For this review, take the finished solid that the model builds, in its own axes (mm). Give positions to 0.01 mm unless a question says otherwise; leave off trailing zeros. Write each loop counter-clockwise with the first axis right and the second up, starting at its lowest first coordinate (ties: lowest second). Pieces come first, ordered by that corner, then holes. Notation, with made-up numbers: M 68.5,7 L 108.5,7 A5 ccw 108.5,16 Z; hole C 78.25,-22.5 d9. An arc over 180 degrees is marked long. Use one line per item in the form item = value. Start each with the question number.
Q1. Consider section A-A on z = -2.75. Write out the cut boundary in (x, y).
Q2. Consider section C-C on y = 2. Write out the cut boundary in (x, z).
Q3. Consider section B-B on x = 31. Write out the cut boundary in (y, z), and give its area (3 significant figures).
Q4. For probe 1 along X at (y, z) = (8, 0); probe 2 along Y at (x, z) = (35, 0), list the stretches that pass through material, from the lowest coordinate up. Write a range as [from, to].
Q5. Clearance check with flat-ended pins moving along their axes: pin 1 Ø6 at (y, z) = (5, 2.5) entering from +X; pin 2 Ø0.6 at (x, y) = (-5.5, 10.5) entering from -Z; pin 3 Ø1.5 at (y, z) = (9, -1) entering from +X. State where each tip first meets the part, or that it passes through.
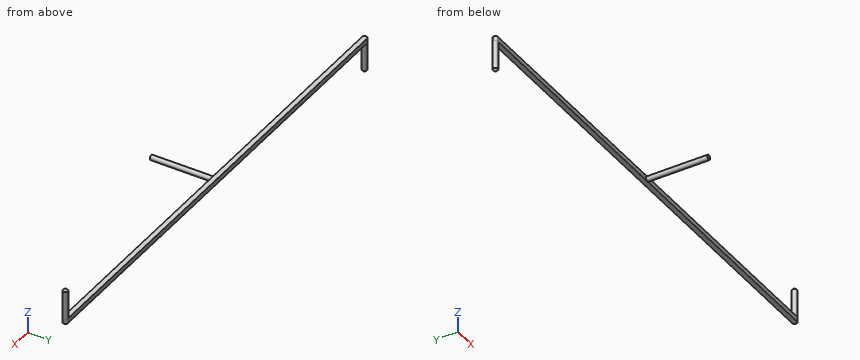
```python
from build123d import *

# Parameters (mm, degrees)
SKETCH_1_R      = 0.4
EXTRUDE_1_DEPTH = 10
SKETCH_2_W      = 80
SKETCH_2_H      = 0.8
EXTRUDE_2_DEPTH = 0.8
FILLET_1_R      = 0.4
SKETCH_3_R      = 0.4
EXTRUDE_3_DEPTH = 5
SKETCH_4_R      = 0.4
EXTRUDE_4_DEPTH = 5
CHAMFER_1_SIZE  = 0.4


with BuildPart() as part:
    # 草图1 → 凸台-拉伸1 (new body)
    with BuildSketch(Plane(origin=(0, 0, 0), x_dir=(1, 0, 0), z_dir=(0, 1, 0))):
        with Locations(Location((0, 0, 0), (0, 0, 270))):
            Circle(SKETCH_1_R)
    extrude(amount=EXTRUDE_1_DEPTH)

    # 草图2 → 凸台-拉伸2 (add)
    with BuildSketch(Plane(origin=(0, 10, 0), x_dir=(1, 0, 0), z_dir=(0, 1, 0))):
        Rectangle(SKETCH_2_W, SKETCH_2_H)
    extrude(amount=EXTRUDE_2_DEPTH)

    # 圆角1
    fillet_1_edges = [part.edges().sort_by_distance(p)[0] for p in [
        (40, 10, 0),
        (40, 10.8, 0),
        (-40, 10, 0),
        (-40, 10.8, 0),
    ]]
    fillet(fillet_1_edges, radius=FILLET_1_R - 0.0001)  # a hair under: the kernel refuses the full size

    # 草图3 → 凸台-拉伸3 (add)
    with BuildSketch(Plane.XY.offset(0.4)):
        with Locations((39.6, 10.4)):
            Circle(SKETCH_3_R)
    extrude(amount=EXTRUDE_3_DEPTH)

    # 草图4 → 凸台-拉伸4 (add)
    with BuildSketch(Plane(origin=(0, 0, -0.4), x_dir=(-1, 0, 0), z_dir=(0, 0, -1))):
        with Locations((39.6, 10.4)):
            Circle(SKETCH_4_R)
    extrude(amount=EXTRUDE_4_DEPTH)

    # 倒角1
    chamfer_1_edges = [part.edges().sort_by_distance(p)[0] for p in [
        (39.2, 10.4, 5.4),
        (-39.2, 10.4, -5.4),
    ]]
    chamfer(chamfer_1_edges, length=CHAMFER_1_SIZE - 0.0001)  # a hair under: the kernel refuses the full size


solid = part.part
```
Working result:
q1.outline = C -39.6,10.4 d0.8
q2.outline = C 0,0 d0.8
q3.outline = M 10,-0.4 L 10.8,-0.4 L 10.8,0.4 L 10,0.4 Z
q3.area = 0.640 mm²
q4.probe_1 = [-0.4, 0.4]
q4.probe_2 = [10, 10.8]
q5.pin_1 = 0.4
q5.pin_2 = -0.4
q5.pin_3 = 0.31
